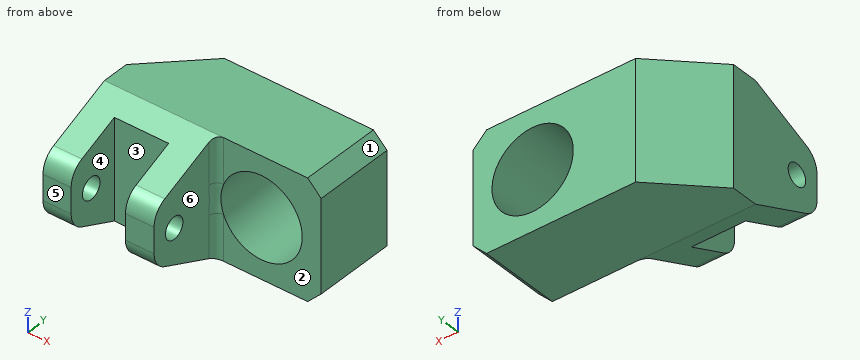
```python
from build123d import *

# Parameters (mm, degrees)
SKETCH_1_W          = 80
SKETCH_1_H          = 44
SKETCH_1_R          = 15
EXTRUDE_1_DEPTH     = 30
CHAMFER_1_SIZE      = 20
SKETCH_2_W          = 41
SKETCH_2_H          = 44
EXTRUDE_2_DEPTH     = 28
SKETCH_3_R          = 4
CUT_EXTRUDE_1_DEPTH = 89.22698
SKETCH_4_W          = 20.030013647
SKETCH_4_H          = 19.701271899
CUT_EXTRUDE_2_DEPTH = 79.74007874
CHAMFER_4_SIZE      = 5
FILLET_1_R          = 3
CUT_EXTRUDE_3_DEPTH = 89.226980059
FILLET_2_R          = 8


with BuildPart() as part:
    # Эскиз1 → Вытянуть1 (new body)
    with BuildSketch(Plane(origin=(0, 0, 0), x_dir=(1, 0, 0), z_dir=(0, 1, 0))):
        with Locations((-18, 0)):
            Rectangle(SKETCH_1_W, SKETCH_1_H)
        with Locations(Location((0, 0, 0), (0, 0, 270))):
            Circle(SKETCH_1_R, mode=Mode.SUBTRACT)
    extrude(amount=EXTRUDE_1_DEPTH)

    # Фаска1
    chamfer_1_edges = [part.edges().sort_by_distance(p)[0] for p in [
        (-58, 30, 0),
    ]]
    chamfer(chamfer_1_edges, length=CHAMFER_1_SIZE)

    # Эскиз2 → Вытянуть2 (add)
    with BuildSketch(Plane.XZ):
        with Locations((-37.5, 0)):
            Rectangle(SKETCH_2_W, SKETCH_2_H)
    extrude(amount=EXTRUDE_2_DEPTH)

    # Эскиз3 → Вырез-Вытянуть1 (cut, through all)
    with BuildSketch(Plane.ZY.offset(58)):
        with Locations((-0.788742376, -18.841346952)):
            Circle(SKETCH_3_R)
    extrude(amount=-CUT_EXTRUDE_1_DEPTH, mode=Mode.SUBTRACT)

    # Эскиз4 → Вырез-Вытянуть2 (cut, through all)
    with BuildSketch(Plane.XY.offset(22)):
        with Locations((-37.59406334, -18.149364051)):
            Rectangle(SKETCH_4_W, SKETCH_4_H)
    extrude(amount=-CUT_EXTRUDE_2_DEPTH, mode=Mode.SUBTRACT)

    # Фаска4
    chamfer_4_edges = [part.edges().sort_by_distance(p)[0] for p in [
        (22, 15, -22),
        (22, 15, 22),
    ]]
    chamfer(chamfer_4_edges, length=CHAMFER_4_SIZE)

    # Скругление1
    fillet_1_edges = [part.edges().sort_by_distance(p)[0] for p in [
        (-17, 0, 0),
    ]]
    fillet(fillet_1_edges, radius=FILLET_1_R)

    # Эскиз5 → Вырез-Вытянуть3 (cut, through all)
    with BuildSketch(Plane.ZY.offset(58)):
        Polygon((-22, 0), (-10, -28), (-22, -28), align=None)
        Polygon((22, -28), (10, -28), (22, 0), align=None)
    extrude(amount=-CUT_EXTRUDE_3_DEPTH, mode=Mode.SUBTRACT)

    # Скругление2
    fillet_2_edges = [part.edges().sort_by_distance(p)[0] for p in [
        (-22.289528258, -28, -10),
        (-52.804535082, -28, -10),
        (-52.804535082, -28, 10),
        (-22.289528258, -28, 10),
    ]]
    fillet(fillet_2_edges, radius=FILLET_2_R)


solid = part.part
```
Read the model definition and answer for the solid it produces. Units are mm, in the model's axes. Face numbers are marked on the shaded views. A direction names the side the tool comes from. Coordinates: 2 decimals unless noted, no trailing zeros. Order: outer loops, then holes, each group sorted by start corner. A loop starts at its lowest first (then second) coordinate and runs counter-clockwise, first axis right, second up. Notation, with made-up numbers: (33.25, 60.25) - (87.25, 60.25) arc R26 cw to (87.25, 77.25) - close; hole circle Ø3 at (-4, 16.25). An arc over 180 degrees is marked (long way). Answer as a JSON object with one key per item and string values. Group by question number.
Item 1: Section B-B (y = 11.5) is taken. Give the vertices of the cut face in (x, z), plus the area to 3 significant figures.
Item 2: A tool of negligible diameter and unlimited length cuts with its end or side. For the marked faces 1, 2 and 3, from which of +Z, -Z, +X, -X, +Y, -Y can it reach the whole face along a straight path? Write none if from no direction.
Item 3: Flat-ended cylindrical pins translate along their axes: P1, Ø3, axis at y = -22, z = -5, coming from the +X side; P2, Ø10, axis at x = -33.5, z = -2, coming from the -Y side; P3, Ø12, axis at x = -14.5, z = -15, coming from the -Y side. Find the tip coordinate at first contact, or state that the pin passes through.
Item 4: Section A-A (x = 14) is taken. Give the vertices of the cut face in (y, z), plus the area to 3 significant figures.
Item 5: Section C-C (z = -16) is taken. Give the vertices of the cut face in (x, y).
Item 6: Section D-D (z = 7) is taken. Give the vertices of the cut face in (x, y), plus the area to 3 significant figures.
Item 7: Consider probe 1 along X at (y, z) = (8, 0); probe 2 along Z at (x, y) = (0, 18); probe 3 along X at (y, z) = (-9.5, 7). Determine where each line is inside the solid, lowest interval first. Write a range as from..to.
Item 8: The mould has two halves that part along X. Classify the marked faces 4, 5 and 6: +X half, -X half, draft (parallel to the pull), parting line (faces both ways), or undercut.
Results are:
{
 "1": {"outline": "(-56.5, -22) - (17, -22) - (22, -17) - (22, 17) - (17, 22) - (-56.5, 22) - close; hole circle Ø30 at (0, 0)", "area": "2,720 mm^2"},
 "2": {"face 1": "+Z, +X, +Y, -Y", "face 2": "+Z, -Z, +X, -Y", "face 3": "+Z, -Z, -Y"},
 "3": {"P1": "stops at x = -17", "P2": "stops at y = -8.3", "P3": "stops at y = -26.38"},
 "4": {"outline": "(0, -22) - (30, -22) - (30, -5.39) - (0, -5.39) - close; (0, 5.39) - (30, 5.39) - (30, 22) - (0, 22) - close", "area": "997 mm^2"},
 "5": {"outline": "(-58, -14) - (-47.61, -14) - (-47.61, -8.3) - (-27.58, -8.3) - (-27.58, -14) - (-17, -14) - (-17, -3) arc R3 cw to (-14, 0) - (22, 0) - (22, 30) - (-38, 30) - (-58, 10) - close"},
 "6": {"outline": "(-58, -27.67) - (-47.61, -27.67) - (-47.61, -8.3) - (-27.58, -8.3) - (-27.58, -27.67) - (-17, -27.67) - (-17, -3) arc R3 cw to (-14, 0) - (-13.27, 0) - (-13.27, 30) - (-38, 30) - (-58, 10) - close; (13.27, 0) - (22, 0) - (22, 30) - (13.27, 30) - close", "area": "2,150 mm^2"},
 "7": {"probe 1": "x = -58..-15, 15..22", "probe 2": "z = -22..-15, 15..22", "probe 3": "x = -58..-47.61, -27.58..-17"},
 "8": {"face 4": "undercut", "face 5": "draft", "face 6": "+X half"}
}
